For this review, use the dimensioned drawing (mm, ordinates from the lowest corner) and the shaded views. Coordinates: 2 decimals unless noted, no trailing zeros. Order: outer loops, then holes, each group sorted by start corner. A loop starts at its lowest first (then second) coordinate and runs counter-clockwise, first axis right, second up. Notation, with made-up numbers: M 62.5,19 L 111.5,19 A12 cw 111.5,24 Z; hole C -4,22.25 d11. An arc over 180 degrees is marked long. One line per item, written item: value.
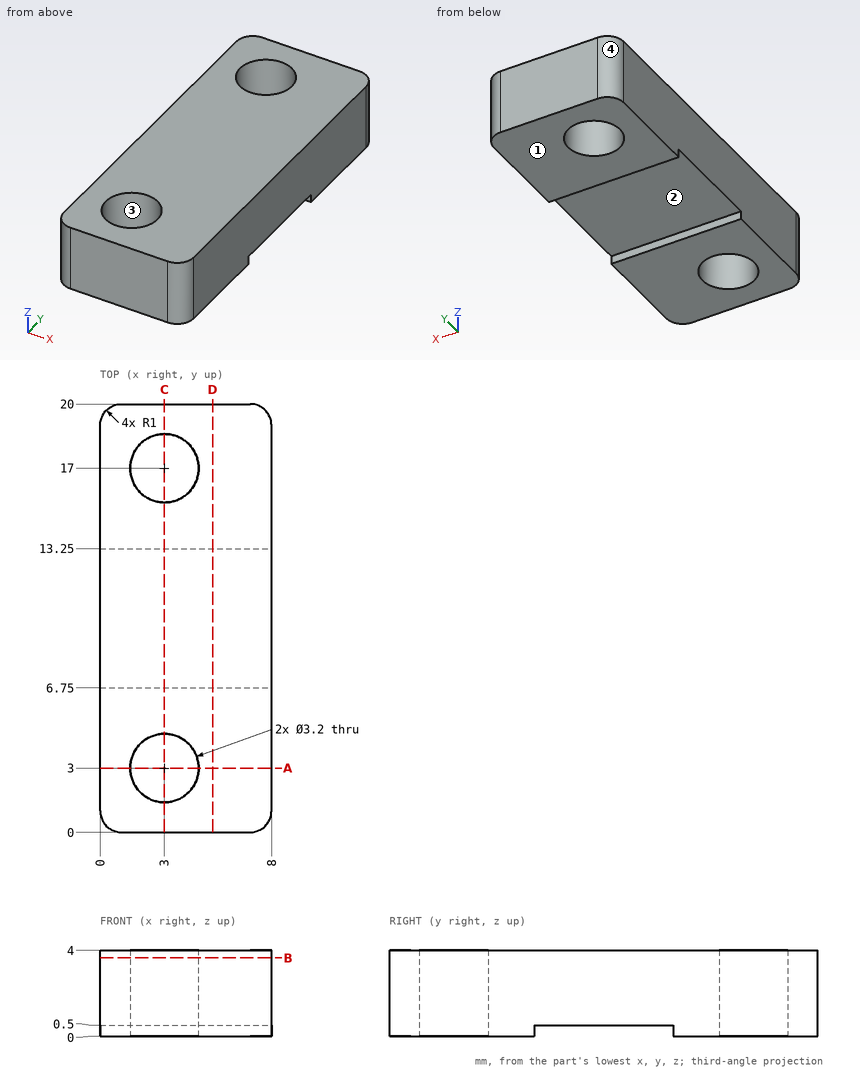
(1) We need section C-C, the plane x = 3. State the section outline as (y, z) points.
Geometry results:
outline: M 0,0 L 1.4,0 L 1.4,4 L 0,4 Z; M 4.6,0 L 6.75,0 L 6.75,0.5 L 13.25,0.5 L 13.25,0 L 15.4,0 L 15.4,4 L 4.6,4 Z; M 18.6,0 L 20,0 L 20,4 L 18.6,4 Z
(2) Insertion check: pin 1 Ø1.9 at (x, y) = (3, 3) entering from -Z. The pin has a flat end and moves straight along its axis. Give the tip position at first contact, or say it passes through.
Geometry results:
pin 1: passes through
(3) We need section B-B, the plane z = 3.65. State the section outline as (x, y) points, plus the area to 3 significant figures.
Geometry results:
outline: M 0,1 A1 ccw 1,0 L 7,0 A1 ccw 8,1 L 8,19 A1 ccw 7,20 L 1,20 A1 ccw 0,19 Z; hole C 3,3 d3.2; hole C 3,17 d3.2
area: 143 mm2
(4) Mouldability with a two-part tool opening along Y and no side actions: class the marked faces 1, 2, 3 and 4 as +Y half, -Y half, draft (parallel to the pull), parting line (faces both ways), or undercut.
Geometry results:
face 1: draft
face 2: undercut
face 3: undercut
face 4: +Y half
(5) We need section A-A, the plane y = 3. State the section outline as (x, z) points.
Geometry results:
outline: M 0,0 L 1.4,0 L 1.4,4 L 0,4 Z; M 4.6,0 L 8,0 L 8,4 L 4.6,4 Z
(6) We need section D-D, the plane x = 5.25. State the section outline as (y, z) points, plus the area to 4 significant figures.
Geometry results:
outline: M 0,0 L 6.75,0 L 6.75,0.5 L 13.25,0.5 L 13.25,0 L 20,0 L 20,4 L 0,4 Z
area: 76.75 mm2
(7) For L1, parallel to Y at x = 3, z = 1.1; L2, parallel to X at y = 3, z = 2.1; L3, parallel to Y at x = 3.5, z = 1.5, list the stretches that pass through material, from the lowest coordinate up.
Geometry results:
L1: y = 0 to 1.4, 4.6 to 15.4, 18.6 to 20
L2: x = 0 to 1.4, 4.6 to 8
L3: y = 0 to 1.48, 4.52 to 15.48, 18.52 to 20
